Autodesk Inventor part; units mm, degrees
ref_plane "YZ Plane" through (0, 0, 0) normal (1, 0, 0) x (0, 1, 0)
ref_plane "XZ Plane" through (0, 0, 0) normal (0, 1, 0) x (-1, 0, 0)
ref_plane "XY Plane" through (0, 0, 0) normal (0, 0, 1) x (1, 0, 0)
sketch "Sketch1" plane through (0, 0, 0) normal (0, 0, 1) x (1, 0, 0)
  line L0 (-75, -12.5) -> (75, -12.5)
  line L1 (75, -12.5) -> (75, 12.5)
  line L2 (75, 12.5) -> (-75, 12.5)
  line L3 (-75, 12.5) -> (-75, -12.5)
  line L4 (-75, -12.5) -> (75, 12.5) construction
  line L5 (75, -12.5) -> (-75, 12.5) construction
  circle A0 centre (-57.5, 0) radius 4.25
  circle A1 centre (0, 0) radius 4.25
  circle A2 centre (57.5, 0) radius 4.25
  line L6 (-57.5, 0) -> (57.5, 0) construction
  dimension "d0" = 150
  dimension "d1" = 25
  dimension "d3" = 115
  dimension "d4" = 8.5
extrude "Extrusion1" add sketch "Sketch1" along normal blind 5
chamfer "Chamfer1" distance 5 angle 45 4 edges at (-75, 12.5, 2.5) (-75, -12.5, 2.5) (75, -12.5, 2.5) (75, 12.5, 2.5)
properties part number "GUIA_DE_AYUDA" material "Steel, Mild, Welded"
For this review, take the finished solid that the model builds, in its own axes (mm). Coordinates: 2 decimals unless noted, no trailing zeros. Loops run counter-clockwise (first coordinate to the right, second up) from the corner with the lowest first, then second, coordinate; pieces in that order, holes last. Notation, with made-up numbers: (-27.5, 21.5) - (-11.5, 21.5) arc R17 ccw to (-11.5, 29.5) - close; hole circle Ø6 at (50.25, 69). An arc over 180 degrees is marked (long way). Use a Markdown table: item, result. Add a question column.
Item 1: We need section B-B (z = 2.15). Give the boundary of the cut face in (x, y), and give its area (3 significant figures).
Item 2: We need section D-D (x = 59.5). Give the boundary of the cut face in (y, z).
Item 3: We need section A-A (y = -2). Give the boundary of the cut face in (x, z).
Item 4: Insertion check: pin 1 Ø7 at (x, y) = (57.5, 0) entering from +Z; pin 2 Ø1.5 at (x, y) = (15.5, -8.5) entering from -Z. Each pin has a flat end and moves straight along its axis. Give the tip position at first contact, or say it passes through.
Item 5: Mouldability with a two-part tool opening along Y and no side actions: class faces 1 (the face through (-75, 0, 2)), 2 (the face through (2.285, -3.584, 2.465)), 3 (the face through (72.5, -10, 2.5)) as pulls with the +Y half, pulls with the -Y half, needs draft (parallel to the pull), parting line crosses it, or undercut.
Item 6: We need section C-C (x = -57.5). Give the boundary of the cut face in (y, z).
Item 7: For line 1 (Y direction, x = 57.5, z = 3.7); line 2 (Y direction, x = -1, z = 0.9); line 3 (X direction, y = -9.25, z = 3.25), list the stretches that pass through material, from the lowest coordinate up.
Results list:
| question | item | result |
|---|---|---|
| 1 | outline | (-75, -7.5) - (-70, -12.5) - (70, -12.5) - (75, -7.5) - (75, 7.5) - (70, 12.5) - (-70, 12.5) - (-75, 7.5) - close; hole circle Ø8.5 at (-57.5, 0); hole circle Ø8.5 at (0, 0); hole circle Ø8.5 at (57.5, 0) |
| 1 | area | 3,530 mm^2 |
| 2 | outline | (-12.5, 0) - (-3.75, 0) - (-3.75, 5) - (-12.5, 5) - close; (3.75, 0) - (12.5, 0) - (12.5, 5) - (3.75, 5) - close |
| 3 | outline | (-75, 0) - (-61.25, 0) - (-61.25, 5) - (-75, 5) - close; (-53.75, 0) - (-3.75, 0) - (-3.75, 5) - (-53.75, 5) - close; (3.75, 0) - (53.75, 0) - (53.75, 5) - (3.75, 5) - close; (61.25, 0) - (75, 0) - (75, 5) - (61.25, 5) - close |
| 4 | pin 1 | passes through |
| 4 | pin 2 | stops at z = 0 |
| 5 | face 1 | needs draft |
| 5 | face 2 | undercut |
| 5 | face 3 | pulls with the -Y half |
| 6 | outline | (-12.5, 0) - (-4.25, 0) - (-4.25, 5) - (-12.5, 5) - close; (4.25, 0) - (12.5, 0) - (12.5, 5) - (4.25, 5) - close |
| 7 | line 1 | y = -12.5 to -4.25, 4.25 to 12.5 |
| 7 | line 2 | y = -12.5 to -4.13, 4.13 to 12.5 |
| 7 | line 3 | x = -73.25 to 73.25 |
